Model file for the job. Use its own axes, mm. Face numbers are marked on the shaded views. A direction names the side the tool comes from. Round coordinates to 2 decimals unless told otherwise and drop trailing zeros. Order: outer loops, then holes, each group sorted by start corner. A loop starts at its lowest first (then second) coordinate and runs counter-clockwise, first axis right, second up. Notation, with made-up numbers: (39, 52.5) - (58, 52.5) arc R29 ccw to (58, 90.5) - close; hole circle Ø5 at (6, 35). An arc over 180 degrees is marked (long way). Put each result on its own line as item: value. Start each with the question number.
Item 1: Saw through at D-D on x = 2.5. List the corners of the cut face in (y, z), plus the area to 3 significant figures.
Item 2: Mould opens along X. For the marked faces 3, 4, 5 and 6 say: pulls with the +X half, pulls with the -X half, needs draft (parallel to the pull), parting line crosses it, or undercut.
Item 3: Saw through at C-C on y = 6.75. List the corners of the cut face in (x, z), plus the area to 3 significant figures.
Item 4: Pin check, flat tips, straight feed: pin 1 Ø8 at (y, z) = (0, 0) entering from -X; pin 2 Ø8 at (x, z) = (4, 5.5) entering from -Y; pin 3 Ø8 at (x, y) = (8.5, 6) entering from +Z; pin 4 Ø4 at (x, y) = (4, -5.5) entering from +Z. Stop position of each tip, or through.
Item 5: Saw through at A-A on y = 0. List the corners of the cut face in (x, z), plus the area to 4 significant figures.
Item 6: Probe probe 1 along X at (y, z) = (-5.5, -4.75); probe 2 along Y at (x, z) = (8.75, 0); probe 3 along Y at (x, z) = (1.25, 5.75). List the from-to ranges inside material, lowest first.
Item 7: Which spindle directions (+Z, -Z, +X, -X, +Y, -Y) get a long thin tool onto all of the face, cutting with end or side? Do the marked faces 1 and 2. Say none if no direction does.
```python
from build123d import *

# Parameters (mm, degrees)
SKETCH1_R           = 8
SKETCH1_R_2         = 2.5
BOSS_EXTRUDE1_DEPTH = 6
SKETCH2_R           = 5.5
SKETCH2_R_2         = 2.5
BOSS_EXTRUDE2_DEPTH = 6
SKETCH3_R           = 8
SKETCH3_R_2         = 2.5
BOSS_EXTRUDE3_DEPTH = 1.5


with BuildPart() as part:
    # Sketch1 → Boss-Extrude1 (new body)
    with BuildSketch(Plane(origin=(0, 0, 0), x_dir=(0, 0, -1), z_dir=(1, 0, 0))):
        Circle(SKETCH1_R)
        Circle(SKETCH1_R_2, mode=Mode.SUBTRACT)
    extrude(amount=BOSS_EXTRUDE1_DEPTH)

    # Sketch2 → Boss-Extrude2 (add)
    with BuildSketch(Plane(origin=(6, 0, 0), x_dir=(0, 0, -1), z_dir=(1, 0, 0))):
        Circle(SKETCH2_R)
        Circle(SKETCH2_R_2, mode=Mode.SUBTRACT)
    extrude(amount=BOSS_EXTRUDE2_DEPTH)

    # Sketch3 → Boss-Extrude3 (add)
    with BuildSketch(Plane(origin=(12, 0, 0), x_dir=(0, 0, -1), z_dir=(1, 0, 0))):
        Circle(SKETCH3_R)
        Circle(SKETCH3_R_2, mode=Mode.SUBTRACT)
    extrude(amount=BOSS_EXTRUDE3_DEPTH)


solid = part.part
```
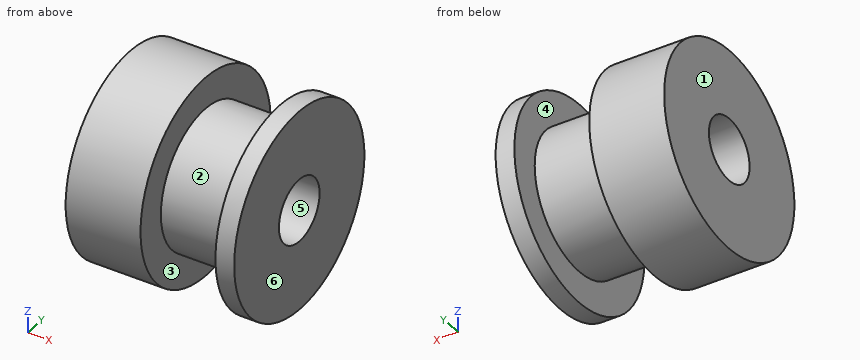
Results found:
1. outline: circle Ø16 at (0, 0); hole circle Ø5 at (0, 0)
1. area: 181 mm²
2. face 3: undercut
2. face 4: undercut
2. face 5: needs draft
2. face 6: pulls with the +X half
3. outline: (0, -4.29) - (6, -4.29) - (6, 4.29) - (0, 4.29) - close; (12, -4.29) - (13.5, -4.29) - (13.5, 4.29) - (12, 4.29) - close
3. area: 64.4 mm²
4. pin 1: stops at x = 0
4. pin 2: stops at y = -7.86
4. pin 3: stops at z = 7.46
4. pin 4: stops at z = 7.19
5. outline: (0, -8) - (6, -8) - (6, -5.5) - (12, -5.5) - (12, -8) - (13.5, -8) - (13.5, -2.5) - (0, -2.5) - close; (0, 2.5) - (13.5, 2.5) - (13.5, 8) - (12, 8) - (12, 5.5) - (6, 5.5) - (6, 8) - (0, 8) - close
5. area: 118.5 mm²
6. probe 1: x = 0 to 6, 12 to 13.5
6. probe 2: y = -5.5 to -2.5, 2.5 to 5.5
6. probe 3: y = -5.56 to 5.56
7. face 1: +Z, -Z, -X, +Y, -Y
7. face 2: none
